```python
from build123d import *

# Parameters (mm, degrees)
F0_R     = 102
F0_R_2   = 2.35
F0_W     = 20
F0_H     = 40
F1_DEPTH = 64


with BuildPart() as f1:
    # F0 (on Top) → F1 (new body)
    with BuildSketch(Plane.XY):
        Circle(F0_R)
        with Locations((-6, -14.2)):
            Circle(F0_R_2, mode=Mode.SUBTRACT)
        with Locations((6, -14.2)):
            Circle(F0_R_2, mode=Mode.SUBTRACT)
        with Locations((-6, 35.2)):
            Circle(F0_R_2, mode=Mode.SUBTRACT)
        with Locations((0, 10.5)):
            Rectangle(F0_W, F0_H, mode=Mode.SUBTRACT)
        with Locations((6, 35.2)):
            Circle(F0_R_2, mode=Mode.SUBTRACT)
    extrude(amount=F1_DEPTH)


solid = f1.part
```
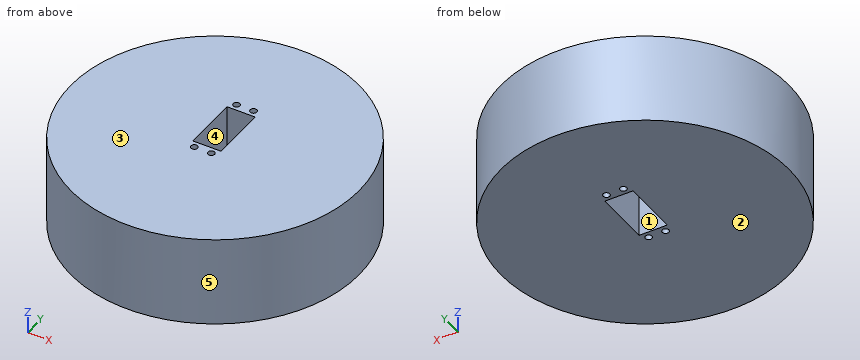
For this review, take the finished solid that the model builds, in its own axes (mm). Face numbers are marked on the shaded views. A direction names the side the tool comes from. Round coordinates to 2 decimals unless told otherwise and drop trailing zeros. Loops run counter-clockwise (first coordinate to the right, second up) from the corner with the lowest first, then second, coordinate; pieces in that order, holes last.
Q1. Add section D-D on x = 45. Write out the cut boundary in (y, z), plus the area to 3 significant figures.
Result sheet:
outline: (-91.54, 0) - (91.54, 0) - (91.54, 64) - (-91.54, 64) - close
area: 11,700 mm2
Q2. Machinability: for the marked faces 1 and 2, which of the approach directions +Z, -Z, +X, -X, +Y, -Y give a long, thin tool a straight path to every point of the face, cutting with its end or side? Answer none if there is none.
Result sheet:
face 1: +Z, -Z
face 2: -Z, +X, -X, +Y, -Y
Q3. Mouldability with a two-part tool opening along X and no side actions: class the marked faces 3, 4 and 5 as +X half, -X half, draft (parallel to the pull), parting line (faces both ways), or undercut.
Result sheet:
face 3: draft
face 4: undercut
face 5: parting line
Q4. Insertion check: pin 1 Ø4 at (x, y) = (-6, 35.2) entering from +Z; pin 2 Ø12 at (x, z) = (-60.5, 49) entering from +Y; pin 3 Ø2 at (x, z) = (-68.5, 12) entering from -Y; pin 4 Ø5 at (x, z) = (-61.5, 38) entering from +Y. Each pin has a flat end and moves straight along its axis. Give the tip position at first contact, or say it passes through.
Result sheet:
pin 1: passes through
pin 2: stops at y = 86.22
pin 3: stops at y = -76.47
pin 4: stops at y = 83.2
Q5. To check wall thickness, follow line 1 along Y through (x, z) = (6, 42); line 2 along Y through (x, z) = (-4.5, 35.5); line 3 along X through (y, z) = (35, 33). State the ranges of each line that lie inside material, in increasing order.
Result sheet:
line 1: y = -101.82 to -16.55, -11.85 to -9.5, 30.5 to 32.85, 37.55 to 101.82
line 2: y = -101.9 to -16.01, -12.39 to -9.5, 30.5 to 33.39, 37.01 to 101.9
line 3: x = -95.81 to -8.34, -3.66 to 3.66, 8.34 to 95.81
Q6. Add section B-B on z = 15.5. Write out the cut boundary in (x, y), plus the area to 3 significant figures.
Result sheet:
outline: circle Ø204 at (0, 0); hole (-10, -9.5) - (10, -9.5) - (10, 30.5) - (-10, 30.5) - close; hole circle Ø4.7 at (-6, -14.2); hole circle Ø4.7 at (-6, 35.2); hole circle Ø4.7 at (6, -14.2); hole circle Ø4.7 at (6, 35.2)
area: 31,800 mm2
Q7. Add section C-C on x = 0. Write out the cut boundary in (y, z).
Result sheet:
outline: (-102, 0) - (-9.5, 0) - (-9.5, 64) - (-102, 64) - close; (30.5, 0) - (102, 0) - (102, 64) - (30.5, 64) - close
Q8. Add section A-A on y = 0. Write out the cut boundary in (x, z), plus the area to 3 significant figures.
Result sheet:
outline: (-102, 0) - (-10, 0) - (-10, 64) - (-102, 64) - close; (10, 0) - (102, 0) - (102, 64) - (10, 64) - close
area: 11,800 mm2
